from build123d import *

# Parameters (mm, degrees)
SKETCH1_W                                           = 100
SKETCH1_H                                           = 70
SKETCH1_R                                           = 5
BOSS_EXTRUDE1_DEPTH                                 = 10
CSK_FOR_M5_COUNTERSUNK_FLAT_HEAD_SCREW1_D           = 5.5
CSK_FOR_M5_COUNTERSUNK_FLAT_HEAD_SCREW1_CSINK_D     = 10.6
CSK_FOR_M5_COUNTERSUNK_FLAT_HEAD_SCREW1_CSINK_ANGLE = 90


with BuildPart() as part:
    # Sketch1 → Boss-Extrude1 (new body)
    with BuildSketch(Plane(origin=(0, 0, 0), x_dir=(1, 0, 0), z_dir=(0, 1, 0))):
        with Locations((50, 35)):
            Rectangle(SKETCH1_W, SKETCH1_H)
        with Locations(Location((50, 35, 0), (0, 0, 270))):
            Circle(SKETCH1_R, mode=Mode.SUBTRACT)
        with BuildLine():
            Line((18.5, 55), (18.5, 15))
            ThreePointArc((18.5, 15), (12.5, 9), (6.5, 15))
            Line((6.5, 15), (6.5, 55))
            ThreePointArc((6.5, 55), (12.5, 61), (18.5, 55))
        make_face(mode=Mode.SUBTRACT)
        with BuildLine():
            Line((93.5, 55), (93.5, 15))
            ThreePointArc((93.5, 15), (87.5, 9), (81.5, 15))
            Line((81.5, 15), (81.5, 55))
            ThreePointArc((81.5, 55), (87.5, 61), (93.5, 55))
        make_face(mode=Mode.SUBTRACT)
    extrude(amount=BOSS_EXTRUDE1_DEPTH)

    # CSK for M5 Countersunk Flat Head Screw1 (through all)
    with Locations(Plane(origin=(0, 10, 0), x_dir=(1, 0, 0), z_dir=(0, 1, 0))):
        with Locations((32.5, 52.5), (67.5, 52.5), (67.5, 17.5), (32.5, 17.5)):
            CounterSinkHole(CSK_FOR_M5_COUNTERSUNK_FLAT_HEAD_SCREW1_D / 2, CSK_FOR_M5_COUNTERSUNK_FLAT_HEAD_SCREW1_CSINK_D / 2, counter_sink_angle=CSK_FOR_M5_COUNTERSUNK_FLAT_HEAD_SCREW1_CSINK_ANGLE)


solid = part.part
Verification items for the finished model (mm, model axes). A direction names the side the tool comes from. Give positions to 0.01 mm unless a question says otherwise; leave off trailing zeros. Write each loop counter-clockwise with the first axis right and the second up, starting at its lowest first coordinate (ties: lowest second). Pieces come first, ordered by that corner, then holes. Notation, with made-up numbers: (61.5, 24) - (110.5, 24) arc R29 ccw to (110.5, 59) - close; hole circle Ø5 at (-5.5, -35.5). An arc over 180 degrees is marked (long way). Answer as CSV lines item,"result". Start each with the question number.
1. Draft check along Z on faces 1 (the face through (100, 5, -35)), 2 (the face through (87.6, 4.9, -9)), 3 (the face through (49, 5, -70)). Enter one of: pulls with the +Z half, pulls with the -Z half, needs draft (parallel to the pull), parting line crosses it, or undercut.
2. Set-up check for faces 4 (the face through (87.4, 4.9, -61)), 5 (the face through (35.4, 7.6, -52.6)): record each of +Z, -Z, +X, -X, +Y, -Y from which the full face is reachable in a straight line by a thin tool's end or side.
3. Thickness scan on line 1 (X direction, y = 2.75, z = -14.5); line 2 (Z direction, x = 67.5, y = 6); line 3 (X direction, y = 2.5, z = -52.5). Record the ranges inside material, lowest first.
4. Depth check by flat-ended pin: pin 1 (5 mm diameter, centred on x = 32.5, z = -17.5, fed in from -Y); pin 2 (6.5 mm diameter, centred on x = 67.5, z = -52.5, fed in from +Y). Enter the tip coordinate at first touch or a pass-through.
5. Sectioned sample at C-C (y = 4.5). Record the boundary of the cut face in (x, z), then the cut area to 3 significant figures.
6. Sectioned sample at A-A (z = -35). Record the boundary of the cut face in (x, y).
7. Sectioned sample at D-D (x = 32.5). Record the boundary of the cut face in (y, z).
8. Sectioned sample at B-B (x = 12.5). Record the boundary of the cut face in (y, z), then the cut area to 3 significant figures.
Derived:
1,face 1,"needs draft"
1,face 2,"undercut"
1,face 3,"pulls with the -Z half"
2,face 4,"+Y, -Y"
2,face 5,"+Y"
3,line 1,"0 to 6.52, 18.48 to 81.52, 93.48 to 100"
3,line 2,"-70 to -55.25, -49.75 to -20.25, -14.75 to 0"
3,line 3,"0 to 6.5, 18.5 to 29.75, 35.25 to 64.75, 70.25 to 81.5, 93.5 to 100"
4,pin 1,"through"
4,pin 2,"y = 7.95"
5,outline,"(0, -70) - (100, -70) - (100, 0) - (0, 0) - close; hole (6.5, -55) arc R6 ccw to (18.5, -55) - (18.5, -15) arc R6 ccw to (6.5, -15) - close; hole circle Ø5.5 at (32.5, -52.5); hole circle Ø5.5 at (32.5, -17.5); hole circle Ø10 at (50, -35); hole circle Ø5.5 at (67.5, -52.5); hole circle Ø5.5 at (67.5, -17.5); hole (81.5, -55) arc R6 ccw to (93.5, -55) - (93.5, -15) arc R6 ccw to (81.5, -15) - close"
5,area,"5,640 mm²"
6,outline,"(0, 0) - (6.5, 0) - (6.5, 10) - (0, 10) - close; (18.5, 0) - (45, 0) - (45, 10) - (18.5, 10) - close; (55, 0) - (81.5, 0) - (81.5, 10) - (55, 10) - close; (93.5, 0) - (100, 0) - (100, 10) - (93.5, 10) - close"
7,outline,"(0, -70) - (10, -70) - (10, -57.8) - (7.45, -55.25) - (0, -55.25) - close; (0, -49.75) - (7.45, -49.75) - (10, -47.2) - (10, -22.8) - (7.45, -20.25) - (0, -20.25) - close; (0, -14.75) - (7.45, -14.75) - (10, -12.2) - (10, 0) - (0, 0) - close"
8,outline,"(0, -70) - (10, -70) - (10, -61) - (0, -61) - close; (0, -9) - (10, -9) - (10, 0) - (0, 0) - close"
8,area,"180 mm²"
